The listing builds one solid part. Answer for the finished solid, in the listing's coordinates (mm). Face numbers are marked on the shaded views. Give positions to 0.01 mm unless a question says otherwise; leave off trailing zeros. Loops run counter-clockwise (first coordinate to the right, second up) from the corner with the lowest first, then second, coordinate; pieces in that order, holes last.
Item 1: The mould has two halves that part along X. Classify the marked faces 1, 2 and 3: pulls with the +X half, pulls with the -X half, needs draft (parallel to the pull), parting line crosses it, or undercut.
Item 2: Each of these flat-tipped pins is pushed along its axis until it touches: pin 1 Ø1 at (y, z) = (17, 97) entering from +X; pin 2 Ø1 at (x, z) = (22, 105) entering from -Y; pin 3 Ø2 at (x, z) = (7.5, 62.5) entering from +Y. Where does it stop, or does it pass through?
Item 3: Consider line 1 along Y through (x, z) = (0, 102.5); line 2 along Z through (x, y) = (-1.5, -26); line 3 along Y through (x, z) = (-30.5, 91.5). Determine where each line is inside the solid, lowest interval first.
Item 4: Section A-A, the plane x = 0 is taken. Give the vertices of the cut face in (y, z), and give its area (3 significant figures).
Item 5: Section D-D, the plane z = 31 is taken. Give the vertices of the cut face in (x, y), and give its area (3 significant figures).
Item 6: Section C-C, the plane z = 78 is taken. Give the vertices of the cut face in (x, y), and give its area (3 significant figures).
from build123d import *

# Parameters (mm, degrees)
CYLINDER003_R     = 35
CYLINDER003_DEPTH = 55
CYLINDER002_R     = 40
CYLINDER002_DEPTH = 55
CYLINDER_R        = 35
CYLINDER_DEPTH    = 8
CYLINDER001_R     = 11
CYLINDER001_DEPTH = 65
FILLET_R          = 2
FILLET001_R       = 1
FILLET002_R       = 1


with BuildPart() as cone:
    # Cone → Cone (revolve)
    with BuildSketch(Plane(origin=(0, 0, 35), x_dir=(1, 0, 0), z_dir=(0, -1, 0))):
        Polygon((0, 0), (6.5, 0), (40, 30), (0, 30), align=None)
    revolve(axis=Axis((0, 0, 35), (0, 0, 1)))


with BuildPart() as cylinder003:
    # Cylinder003 → Cylinder003 (new body)
    with BuildSketch(Plane.XY.offset(69)):
        Circle(CYLINDER003_R)
    extrude(amount=CYLINDER003_DEPTH)


with BuildPart() as cut:
    # Cylinder002 → Cylinder002 (new body)
    with BuildSketch(Plane.XY.offset(65)):
        Circle(CYLINDER002_R)
    extrude(amount=CYLINDER002_DEPTH)

    # Cut: cut Cylinder003
    add(cylinder003.part, mode=Mode.SUBTRACT)


with BuildPart() as cylinder:
    # Cylinder → Cylinder (new body)
    with BuildSketch(Plane.XY):
        Circle(CYLINDER_R)
    extrude(amount=CYLINDER_DEPTH)


with BuildPart() as fillet002:
    # Cylinder001 → Cylinder001 (new body)
    with BuildSketch(Plane.XY):
        Circle(CYLINDER001_R)
    extrude(amount=CYLINDER001_DEPTH)

    # Fusion: union Cylinder
    add(cylinder.part)

    # Fusion001: union Cut
    add(cut.part)

    # Fusion002: union Cone
    add(cone.part)

    # Fillet
    fillet_edges = [fillet002.edges().sort_by_distance(p)[0] for p in [
        (-35, 0, 8),
    ]]
    fillet(fillet_edges, radius=FILLET_R)

    # Fillet001
    fillet001_edges = [fillet002.edges().sort_by_distance(p)[0] for p in [
        (-40, 0, 120),
    ]]
    fillet(fillet001_edges, radius=FILLET001_R)

    # Fillet002
    fillet002_edges = [fillet002.edges().sort_by_distance(p)[0] for p in [
        (-35, 0, 120),
    ]]
    fillet(fillet002_edges, radius=FILLET002_R)


solid = fillet002.part
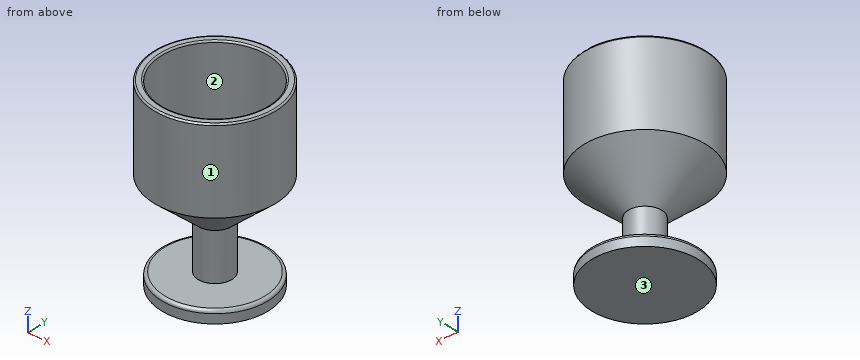
Worked answers:
1. face 1: parting line crosses it
1. face 2: undercut
1. face 3: needs draft
2. pin 1: stops at x = 36.44
2. pin 2: stops at y = -33.73
2. pin 3: stops at y = 37.6
3. line 1: y = -40 to -35, 35 to 40
3. line 2: z = 0 to 8, 52.5 to 69
3. line 3: y = -25.88 to -17.17, 17.17 to 25.88
4. outline: (-40, 65) - (-11, 39.03) - (-11, 8) - (-33, 8) arc R2 ccw to (-35, 6) - (-35, 0) - (35, 0) - (35, 6) arc R2 ccw to (33, 8) - (11, 8) - (11, 39.03) - (40, 65) - (40, 119) arc R1 ccw to (39, 120) - (36, 120) arc R1 ccw to (35, 119) - (35, 69) - (-35, 69) - (-35, 119) arc R1 ccw to (-36, 120) - (-39, 120) arc R1 ccw to (-40, 119) - close
4. area: 3,390 mm2
5. outline: circle Ø22 at (0, 0)
5. area: 380 mm2
6. outline: circle Ø80 at (0, 0); hole circle Ø70 at (0, 0)
6. area: 1,180 mm2
